Read the model definition and answer for the solid it produces. Units are mm, in the model's axes. Round coordinates to 2 decimals unless told otherwise and drop trailing zeros. Loops run counter-clockwise (first coordinate to the right, second up) from the corner with the lowest first, then second, coordinate; pieces in that order, holes last. Notation, with made-up numbers: (56.5, 46) -> (71.5, 46) arc R29 ccw to (71.5, 80) -> close; hole circle Ø8 at (75, -13.5). An arc over 180 degrees is marked (long way). Put each result on its own line as item: value.
from build123d import *

# Parameters (mm, degrees)
SKETCH2_W               = 168.275
SKETCH2_H               = 177.8
SKETCH2_R               = 3.048
SKETCH2_R_2             = 2.413
SKETCH2_R_3             = 1.4224
SKETCH2_R_4             = 3.429
BOSS_EXTRUDE2_DEPTH     = 12.7
CUT_EXTRUDE1_DEPTH      = 1
CUT_EXTRUDE1_DEPTH_BACK = 13.7
FILLET1_R               = 5.08


with BuildPart() as part:
    # Sketch2 → Boss-Extrude2 (new body)
    with BuildSketch(Plane(origin=(0, 0, 0), x_dir=(1, 0, 0), z_dir=(0, 1, 0))):
        with Locations((84.1375, 88.9)):
            Rectangle(SKETCH2_W, SKETCH2_H)
        with Locations((84.1375, 101.6)):
            Circle(SKETCH2_R, mode=Mode.SUBTRACT)
        with Locations((96.8375, 88.9)):
            Circle(SKETCH2_R, mode=Mode.SUBTRACT)
        with Locations((84.1375, 76.2)):
            Circle(SKETCH2_R, mode=Mode.SUBTRACT)
        with Locations((71.4375, 88.9)):
            Circle(SKETCH2_R, mode=Mode.SUBTRACT)
        with Locations((32.8295, 117.475)):
            Circle(SKETCH2_R_2, mode=Mode.SUBTRACT)
        with Locations((135.4455, 117.475)):
            Circle(SKETCH2_R, mode=Mode.SUBTRACT)
        with Locations((135.4455, 60.325)):
            Circle(SKETCH2_R, mode=Mode.SUBTRACT)
        with Locations((32.8295, 60.325)):
            Circle(SKETCH2_R_2, mode=Mode.SUBTRACT)
        with Locations((6.35, 171.45)):
            Circle(SKETCH2_R_3, mode=Mode.SUBTRACT)
        with Locations((161.925, 171.45)):
            Circle(SKETCH2_R_3, mode=Mode.SUBTRACT)
        with Locations((161.925, 6.35)):
            Circle(SKETCH2_R_3, mode=Mode.SUBTRACT)
        with Locations((6.35, 6.35)):
            Circle(SKETCH2_R_3, mode=Mode.SUBTRACT)
        with Locations((31.251071429, 33.02)):
            Circle(SKETCH2_R_3, mode=Mode.SUBTRACT)
        with Locations((137.023928571, 33.02)):
            Circle(SKETCH2_R_3, mode=Mode.SUBTRACT)
        with Locations((84.1375, 119.0625)):
            Circle(SKETCH2_R_4, mode=Mode.SUBTRACT)
        with Locations((114.3, 88.9)):
            Circle(SKETCH2_R_4, mode=Mode.SUBTRACT)
        with Locations((84.1375, 58.7375)):
            Circle(SKETCH2_R_4, mode=Mode.SUBTRACT)
        with Locations((53.975, 88.9)):
            Circle(SKETCH2_R_4, mode=Mode.SUBTRACT)
        with Locations((31.149471429, 145.2372)):
            Circle(SKETCH2_R_3, mode=Mode.SUBTRACT)
        with Locations((137.125528571, 145.161)):
            Circle(SKETCH2_R_3, mode=Mode.SUBTRACT)
    extrude(amount=BOSS_EXTRUDE2_DEPTH)

    # Sketch3 → Cut-Extrude1 (cut, two sides)
    with BuildSketch(Plane(origin=(0, 12.7, 0), x_dir=(1, 0, 0), z_dir=(0, 1, 0))) as cut_extrude1_sk:
        Polygon((0, 165.1), (0, 76.2), (25.4, 76.2), (25.4, 132.589482542), align=None)
    extrude(amount=CUT_EXTRUDE1_DEPTH, mode=Mode.SUBTRACT)
    extrude(cut_extrude1_sk.sketch, amount=-CUT_EXTRUDE1_DEPTH_BACK, mode=Mode.SUBTRACT)

    # Fillet1
    fillet1_edges = [part.edges().sort_by_distance(p)[0] for p in [
        (0, 6.35, -165.1),
        (25.4, 6.35, -132.589482542),
        (25.4, 6.35, -76.2),
        (0, 6.35, -76.2),
        (0, 6.35, -177.8),
        (168.275, 6.35, -177.8),
        (168.275, 6.35, 0),
        (0, 6.35, 0),
    ]]
    fillet(fillet1_edges, radius=FILLET1_R)


solid = part.part
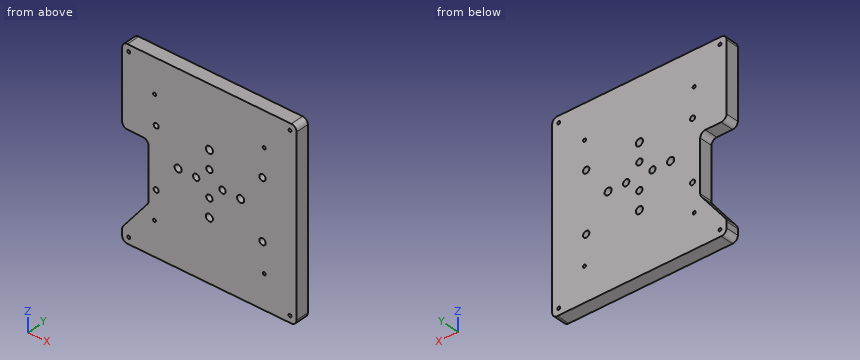
Item 1: The part is cut by section C-C (y = 7.25). State how many separate pieces and enclosed holes the cut face has, then the cut area to 3 significant figures.
Derived:
separate pieces: 1
enclosed holes: 20
area: 27,600 mm^2
Item 2: Flat-ended cylindrical pins translate along their axes: pin 1 Ø2.5 at (x, z) = (161.925, -6.35) entering from +Y; pin 2 Ø4 at (y, z) = (11, -80) entering from -X. Find the tip coordinate at first contact, or state that the pin passes through.
Derived:
pin 1: passes through
pin 2: stops at x = 24.2
Item 3: The part is cut by section B-B (z = -88.9). Determine the outline of the cut face in (x, y) (1 decimal), then the cut area to 3 significant figures.
Derived:
outline: (25.4, 0) -> (50.5, 0) -> (50.5, 12.7) -> (25.4, 12.7) -> close; (57.4, 0) -> (68.4, 0) -> (68.4, 12.7) -> (57.4, 12.7) -> close; (74.5, 0) -> (93.8, 0) -> (93.8, 12.7) -> (74.5, 12.7) -> close; (99.9, 0) -> (110.9, 0) -> (110.9, 12.7) -> (99.9, 12.7) -> close; (117.7, 0) -> (168.3, 0) -> (168.3, 12.7) -> (117.7, 12.7) -> close
area: 1,490 mm^2
Item 4: Find the intervals of material crossed by line 1 along X through (y, z) = (9.5, -88.9) (1 decimal); line 2 along X through (y, z) = (3, -171.45) (3 decimals); line 3 along X through (y, z) = (1.25, -145.5) (3 decimals), in increasing order.
Derived:
line 1: x = 25.4 to 50.5, 57.4 to 68.4, 74.5 to 93.8, 99.9 to 110.9, 117.7 to 168.3
line 2: x = 0 to 4.928, 7.772 to 160.503, 163.347 to 168.275
line 3: x = 15.313 to 29.752, 32.547 to 135.744, 138.507 to 168.275
Item 5: The part is cut by section A-A (x = 114.3). Determine the outline of the cut face in (y, z).
Derived:
outline: (0, -177.8) -> (12.7, -177.8) -> (12.7, -92.33) -> (0, -92.33) -> close; (0, -85.47) -> (12.7, -85.47) -> (12.7, 0) -> (0, 0) -> close
